from build123d import *

# Parameters (mm, degrees)
BOSS_EXTRUDE1_DEPTH = 880
CHAMFER1_SIZE       = 50.8
CHAMFER1_SIZE2      = 71.842048969
SKETCH3_W           = 750
SKETCH3_H           = 50
CUT_EXTRUDE1_DEPTH  = 2.5
SKETCH4_R           = 23.5
CUT_EXTRUDE2_DEPTH  = 11.9
SHELL1_START        = -14.4
SHELL1_OUTLINE_W    = 62.4
SHELL1_OUTLINE_H    = 765
SHELL1_OUTLINE_R    = 23.5
SHELL1_DEPTH        = 4.4
SHELL1_START_2      = 7.5
SHELL1_2_DEPTH      = 865
SHELL1_3_DEPTH      = 50
SHELL1_START_3      = 822.5
SHELL1_4_DEPTH      = 50


with BuildPart() as part:
    # Sketch1 → Boss-Extrude1 (new body)
    with BuildSketch(Plane.XY):
        Polygon((-70.710678119, 70.710678119), (-70.710678119, -70.710678119), (0, 0), align=None)
    extrude(amount=BOSS_EXTRUDE1_DEPTH)

    # Chamfer1
    chamfer1_edges = [part.edges().sort_by_distance(p)[0] for p in [
        (-70.710678119, -70.710678119, 440),
    ]]
    chamfer1_side = [part.faces().sort_by_distance(p)[0] for p in [
        (-35.355339059, -35.355339059, 440),
    ]]
    chamfer(chamfer1_edges, length=CHAMFER1_SIZE, length2=CHAMFER1_SIZE2, reference=chamfer1_side[0])

    # Sketch3 → Cut-Extrude1 (cut)
    with BuildSketch(Plane(origin=(0, 0, 0), x_dir=(0, 0, -1), z_dir=(0.7071067811865493, 0.7071067811865457, 0))):
        with Locations((-440, 37.4)):
            Rectangle(SKETCH3_W, SKETCH3_H)
    extrude(amount=-CUT_EXTRUDE1_DEPTH, mode=Mode.SUBTRACT)

    # Sketch4 → Cut-Extrude2 (cut)
    with BuildSketch(Plane(origin=(-1.767766953, -1.767766953, 0), x_dir=(0, 0, -1), z_dir=(0.7071067811865652, 0.7071067811865298, 0))):
        with Locations(Location((-440, 37.4, 0), (0, 0, 90))):
            Circle(SKETCH4_R)
        with Locations(Location((-490, 37.4, 0), (0, 0, 90))):
            Circle(SKETCH4_R)
        with Locations(Location((-540, 37.4, 0), (0, 0, 90))):
            Circle(SKETCH4_R)
        with Locations(Location((-590, 37.4, 0), (0, 0, 90))):
            Circle(SKETCH4_R)
        with Locations(Location((-640, 37.4, 0), (0, 0, 90))):
            Circle(SKETCH4_R)
        with Locations(Location((-690, 37.4, 0), (0, 0, 90))):
            Circle(SKETCH4_R)
        with Locations(Location((-740, 37.4, 0), (0, 0, 90))):
            Circle(SKETCH4_R)
        with Locations(Location((-790, 37.4, 0), (0, 0, 90))):
            Circle(SKETCH4_R)
        with Locations(Location((-390, 37.4, 0), (0, 0, 90))):
            Circle(SKETCH4_R)
        with Locations(Location((-340, 37.4, 0), (0, 0, 90))):
            Circle(SKETCH4_R)
        with Locations(Location((-290, 37.4, 0), (0, 0, 90))):
            Circle(SKETCH4_R)
        with Locations(Location((-240, 37.4, 0), (0, 0, 90))):
            Circle(SKETCH4_R)
        with Locations(Location((-190, 37.4, 0), (0, 0, 90))):
            Circle(SKETCH4_R)
        with Locations(Location((-140, 37.4, 0), (0, 0, 90))):
            Circle(SKETCH4_R)
        with Locations(Location((-90, 37.4, 0), (0, 0, 90))):
            Circle(SKETCH4_R)
    extrude(amount=-CUT_EXTRUDE2_DEPTH, mode=Mode.SUBTRACT)

    # Shell1: read off the stored shape, not the designer's step
    # Shell1 outline → Shell1 (cut)
    with BuildSketch(Plane(origin=(0, 0, 0), x_dir=(0.7071067811865474, -0.7071067811865477, 0), z_dir=(0.7071067811865476, 0.7071067811865476, 0)).offset(SHELL1_START)):
        with Locations((-38.7, -440)):
            Rectangle(SHELL1_OUTLINE_W, SHELL1_OUTLINE_H)
        with Locations((-37.4, -790)):
            Circle(SHELL1_OUTLINE_R, mode=Mode.SUBTRACT)
        with Locations((-37.4, -740)):
            Circle(SHELL1_OUTLINE_R, mode=Mode.SUBTRACT)
        with Locations((-37.4, -690)):
            Circle(SHELL1_OUTLINE_R, mode=Mode.SUBTRACT)
        with Locations((-37.4, -640)):
            Circle(SHELL1_OUTLINE_R, mode=Mode.SUBTRACT)
        with Locations((-37.4, -590)):
            Circle(SHELL1_OUTLINE_R, mode=Mode.SUBTRACT)
        with Locations((-37.4, -540)):
            Circle(SHELL1_OUTLINE_R, mode=Mode.SUBTRACT)
        with Locations((-37.4, -490)):
            Circle(SHELL1_OUTLINE_R, mode=Mode.SUBTRACT)
        with Locations((-37.4, -440)):
            Circle(SHELL1_OUTLINE_R, mode=Mode.SUBTRACT)
        with Locations((-37.4, -390)):
            Circle(SHELL1_OUTLINE_R, mode=Mode.SUBTRACT)
        with Locations((-37.4, -340)):
            Circle(SHELL1_OUTLINE_R, mode=Mode.SUBTRACT)
        with Locations((-37.4, -290)):
            Circle(SHELL1_OUTLINE_R, mode=Mode.SUBTRACT)
        with Locations((-37.4, -240)):
            Circle(SHELL1_OUTLINE_R, mode=Mode.SUBTRACT)
        with Locations((-37.4, -190)):
            Circle(SHELL1_OUTLINE_R, mode=Mode.SUBTRACT)
        with Locations((-37.4, -140)):
            Circle(SHELL1_OUTLINE_R, mode=Mode.SUBTRACT)
        with Locations((-37.4, -90)):
            Circle(SHELL1_OUTLINE_R, mode=Mode.SUBTRACT)
    extrude(amount=SHELL1_DEPTH, mode=Mode.SUBTRACT)

    # Shell1 2 outline → Shell1 2 (cut)
    with BuildSketch(Plane.XY.offset(SHELL1_START_2)):
        Polygon((-54.730064864, 44.123463146), (-63.210678119, 52.604076401), (-63.210678119, 4.237972568), (-34.789653634, -24.183051917), (-15.485638508, -4.87903679), (-59.609101654, 39.244426356), align=None)
    extrude(amount=SHELL1_2_DEPTH, mode=Mode.SUBTRACT)

    # Shell1 3 outline → Shell1 3 (cut)
    with BuildSketch(Plane.XY.offset(SHELL1_START_2)):
        Polygon((-10.606601718, 0), (-54.730064864, 44.123463146), (-59.609101654, 39.244426356), (-15.485638508, -4.87903679), align=None)
    extrude(amount=SHELL1_3_DEPTH, mode=Mode.SUBTRACT)

    # Shell1 4 outline → Shell1 4 (cut)
    with BuildSketch(Plane.XY.offset(SHELL1_START_3)):
        Polygon((-10.606601718, 0), (-54.730064864, 44.123463146), (-59.609101654, 39.244426356), (-15.485638508, -4.87903679), align=None)
    extrude(amount=SHELL1_4_DEPTH, mode=Mode.SUBTRACT)


solid = part.part
Work out the finished part from the listing and answer in its coordinate system (mm). A direction names the side the tool comes from. Give positions to 0.01 mm unless a question says otherwise; leave off trailing zeros. Loops run counter-clockwise (first coordinate to the right, second up) from the corner with the lowest first, then second, coordinate; pieces in that order, holes last. Notation, with made-up numbers: (68.25, 25.25) -> (76.25, 25.25) arc R33 ccw to (76.25, 59.25) -> close; hole circle Ø7 at (56, -6). An arc over 180 degrees is marked (long way). Use a Markdown table: item, result. Add a question column.
1) The part is cut by section C-C, the plane y = 27. Count the separate pieces of the cut face and the enclosed holes in it, plus the area to 3 significant figures.
2) The part is cut by section B-B, the plane y = 63. Determine the outline of the cut face in (x, z), plus the area to 3 significant figures.
3) Which of the six approach directions +Z, -Z, +X, -X, +Y, -Y give full straight-line access (tool end or side, diameter ignored) to faces 4 (the flat face through (-44, 19, 880)), 5 (the flat face through (-49.2, -9.77, 433.94))?
4) Consider line 1 along Z through (x, y) = (-11, 8); line 2 along Z through (x, y) = (-39, -19); line 3 along Y through (x, z) = (-55.5, 308). Determine where each line is inside the solid, lowest interval first.
5) For a pull along X with two mould halves and no side action, classify faces 1 (the cylindrical face through (-46.18, 37.41, 81)), 2 (the flat face through (-18, -18, 434)), 3 (the flat face through (-44, 19, 0)) as +X half, -X half, draft (parallel to the pull), parting line (faces both ways), or undercut.
6) Each of these flat-tipped pins is pushed along its axis until it touches: P1, Ø10, axis at y = 58, z = 698.5, coming from the +X side; P2, Ø1, axis at y = 25.5, z = 652.5, coming from the +X side; P3, Ø1, axis at x = -25.5, z = 758.5, coming from the -Y side. Where does it stop, or does it pass through?
7) The part is cut by section D-D, the plane z = 448.5. Determine the outline of the cut face in (x, y).
8) The part is cut by section A-A, the plane z = 224. Determine the outline of the cut face in (x, y).
Reported:
| question | item | result |
|---|---|---|
| 1 | separate pieces | 15 |
| 1 | enclosed holes | 0 |
| 1 | area | 9,270 mm^2 |
| 2 | outline | (-70.71, 0) -> (-63, 0) -> (-63, 880) -> (-70.71, 880) -> close |
| 2 | area | 6,790 mm^2 |
| 3 | face 4 | +Z, +X, -X, +Y, -Y |
| 3 | face 5 | none |
| 4 | line 1 | z = 0 to 65, 815 to 880 |
| 4 | line 2 | z = 0 to 7.5, 872.5 to 880 |
| 4 | line 3 | y = -14.08 to -3.47, 41.36 to 43.35, 44.89 to 55.5 |
| 5 | face 1 | undercut |
| 5 | face 2 | +X half |
| 5 | face 3 | draft |
| 6 | P1 | stops at x = -53 |
| 6 | P2 | stops at x = -63.21 |
| 6 | P3 | stops at y = -26 |
| 7 | outline | (-70.71, 1.13) -> (-34.79, -34.79) -> (0, 0) -> (-8.77, 8.77) -> (-10.54, 7) -> (-12.72, 9.19) -> (-18.02, 3.88) -> (-12.37, -1.77) -> (-34.79, -24.18) -> (-63.21, 4.24) -> (-63.21, 52.6) -> (-54.73, 44.12) -> (-56.5, 42.36) -> (-49.01, 34.87) -> (-43.71, 40.17) -> (-45.89, 42.36) -> (-44.12, 44.12) -> (-70.71, 70.71) -> close |
| 8 | outline | (-70.71, 1.13) -> (-34.79, -34.79) -> (0, 0) -> (-8.77, 8.77) -> (-10.54, 7) -> (-16.04, 12.51) -> (-21.35, 7.2) -> (-12.37, -1.77) -> (-34.79, -24.18) -> (-63.21, 4.24) -> (-63.21, 52.6) -> (-54.73, 44.12) -> (-56.5, 42.36) -> (-45.69, 31.55) -> (-40.38, 36.85) -> (-45.89, 42.36) -> (-44.12, 44.12) -> (-70.71, 70.71) -> close |
